```python
from build123d import *

# Parameters (mm, degrees)
SKETCH1_R           = 3
BOSS_EXTRUDE1_DEPTH = 6
FILLET1_R           = 3
CUT_EXTRUDE1_DEPTH  = 33.86335345
CUT_EXTRUDE2_DEPTH  = 23
SKETCH2_4_R         = 2
CUT_EXTRUDE3_DEPTH  = 3
CUT_EXTRUDE4_DEPTH  = 29.930952356


with BuildPart() as part:
    # Sketch1 → Boss-Extrude1 (new, symmetric)
    with BuildSketch(Plane(origin=(0, 0, 0), x_dir=(0, 0, -1), z_dir=(1, 0, 0))):
        with BuildLine():
            Line((-15, 12), (15, 12))
            Line((15, 12), (15, -12))
            Line((15, -12), (-7, -12))
            ThreePointArc((-7, -12), (-8.996142529, -4.664095019), (-15, 0))
            Line((-15, 0), (-15, 12))
        make_face()
        with Locations((-3, -8)):
            Circle(SKETCH1_R, mode=Mode.SUBTRACT)
        with Locations((10, -8)):
            Circle(SKETCH1_R, mode=Mode.SUBTRACT)
    extrude(amount=BOSS_EXTRUDE1_DEPTH, both=True)

    # Fillet1
    fillet1_edges = [part.edges().sort_by_distance(p)[0] for p in [
        (0, -12, -15),
        (0, -12, 7),
        (0, 0, 15),
    ]]
    fillet(fillet1_edges, radius=FILLET1_R)

    # Sketch2 → Cut-Extrude1 (cut, through all)
    with BuildSketch(Plane.XY.offset(15)):
        with BuildLine():
            ThreePointArc((2, 5.278746099), (1.414213562, 6.692959662), (0, 7.278746099))
            Line((0, 7.278746099), (0, 3.278746099))
            ThreePointArc((0, 3.278746099), (1.414213562, 3.864532537), (2, 5.278746099))
        make_face()
        with BuildLine():
            Line((0, 3.278746099), (0, 7.278746099))
            ThreePointArc((0, 7.278746099), (-2, 5.278746099), (0, 3.278746099))
        make_face()
    extrude(amount=-CUT_EXTRUDE1_DEPTH, mode=Mode.SUBTRACT)

    # Sketch2_3 → Cut-Extrude2 (cut)
    with BuildSketch(Plane.XY.offset(15)):
        Polygon((0, 7.746538635), (0, 12), (-3.25, 12), (-4, 7.746538635), align=None)
        Polygon((3.25, 12), (0, 12), (0, 7.746538635), (4, 7.746538635), align=None)
    extrude(amount=-CUT_EXTRUDE2_DEPTH, mode=Mode.SUBTRACT)

    # Sketch2_4 → Cut-Extrude3 (cut)
    # profile 1 of 2: a face of its own
    with BuildSketch(Plane.XY.offset(15)):
        Polygon((3.25, 12), (-3.25, 12), (-4, 7.746538635), (4, 7.746538635), align=None)
    # profile 2 of 2: a face of its own
    with BuildSketch(Plane.XY.offset(15)):
        with BuildLine():
            Line((4, 7.746538635), (-4, 7.746538635))
            ThreePointArc((-4, 7.746538635), (0, 0.578746099), (4, 7.746538635))
        make_face()
        with Locations((0, 5.278746099)):
            Circle(SKETCH2_4_R, mode=Mode.SUBTRACT)
    extrude(amount=-CUT_EXTRUDE3_DEPTH, mode=Mode.SUBTRACT)

    # Sketch3 → Cut-Extrude4 (cut, through all)
    with BuildSketch(Plane(origin=(0, 12, 0), x_dir=(1, 0, 0), z_dir=(0, 1, 0))):
        with BuildLine():
            ThreePointArc((-6, 15), (0, 13.649110641), (6, 15))
            Line((6, 15), (-6, 15))
        make_face()
    extrude(amount=-CUT_EXTRUDE4_DEPTH, mode=Mode.SUBTRACT)


solid = part.part
```
CAD build for the part. Positions are in the model's coordinates, mm. A direction names the side the tool comes from. Give positions to 0.01 mm unless a question says otherwise; leave off trailing zeros. Order: outer loops, then holes, each group sorted by start corner. A loop starts at its lowest first (then second) coordinate and runs counter-clockwise, first axis right, second up.
(1) Saw through at C-C, the plane z = -4.5. Give the cut face in (x, y), then the cut area to 3 significant figures.
(2) Drill centre lines: L1, parallel to Y at x = -0.5, z = -10; L2, parallel to Z at x = 1.5, y = -7; L3, parallel to Z at x = -4.5, y = -9.25. Where is each one in solid material? Low to high.
(3) Saw through at A-A, the plane z = 3. Give the cut face in (x, y).
(4) Mould opens along Z. For faces 1 (the cylindrical face through (-0.08, -5.47, -11.61)), 2 (the cylindrical face through (-0.08, -11.73, -13.24)), 3 (the flat face through (-5, 7, 15)) say: released by +Z, released by -Z, zero draft, split by the parting line, or undercut.
(5) Tool access for faces 4 (the cylindrical face through (-0.14, 0.58, 13.52)), 5 (the cylindrical face through (0.08, 0.09, 14.35)): list every direction of +Z, -Z, +X, -X, +Y, -Y with a clear straight run to the whole face (end or side of a thin tool).
(6) Flat gauge pins, fed straight in: pin 1 (1 mm diameter, centred on x = -0.5, y = 3.5, fed in from +Z); pin 2 (2 mm diameter, centred on x = 1, y = 10.5, fed in from +Z); pin 3 (6.5 mm diameter, centred on x = -0.5, z = 2, fed in from +Y); pin 4 (1.5 mm diameter, centred on x = -1.5, y = 7.5, fed in from -Z). Where does each tip first touch, or does it go through?
(7) Saw through at B-B, the plane x = 0.5. Give the cut face in (y, z), then the cut area to 3 significant figures.
(8) Saw through at D-D, the plane y = -8. Give the cut face in (x, z), then the cut area to 3 significant figures.
Results found:
1. outline: (-6, -12) - (6, -12) - (6, 12) - (3.25, 12) - (4, 7.75) - (-4, 7.75) - (-3.25, 12) - (-6, 12) - close; hole circle Ø4 at (0, 5.28)
1. area: 245 mm2
2. L1: y = -12 to -11, -5 to 3.34, 7.22 to 12
2. L2: z = -13.73 to -12.83, -7.17 to 0.17, 5.83 to 7.79
2. L3: z = -14.39 to -12.73, -7.27 to 0.27, 5.73 to 7.16
3. outline: (-6, -12) - (6, -12) - (6, -11) - (-6, -11) - close; (-6, -5) - (6, -5) - (6, 12) - (3.25, 12) - (4, 7.75) - (-4, 7.75) - (-3.25, 12) - (-6, 12) - close; hole circle Ø4 at (0, 5.28)
4. face 1: undercut
4. face 2: released by -Z
4. face 3: released by +Z
5. face 4: +Z
5. face 5: +Z, +X, -X, -Y
6. pin 1: stops at z = 12
6. pin 2: stops at z = -8
6. pin 3: stops at y = 12
6. pin 4: stops at z = -13.83
7. outline: (-12, -12) arc R3 ccw to (-11.5, -13.66) - (3.34, -13.66) - (3.34, 12) - (0.61, 12) - (0.61, 14.68) arc R3 ccw to (-0.7, 13.4) arc R12 cw to (-9.46, 7.13) arc R3 ccw to (-12, 4.16) - close; (7.22, -13.66) - (12, -13.66) - (12, -8) - (7.75, -8) - (7.75, 12) - (7.22, 12) - close; hole circle Ø6 at (-8, -10); hole circle Ø6 at (-8, 3)
7. area: 339 mm2
8. outline: (-6, -15) arc R14 cw to (6, -15) - (6, -13) - (-6, -13) - close; (-6, -7) - (6, -7) - (6, 0) - (-6, 0) - close; (-6, 6) - (6, 6) - (6, 7.45) - (-6, 7.45) - close
8. area: 114 mm2
